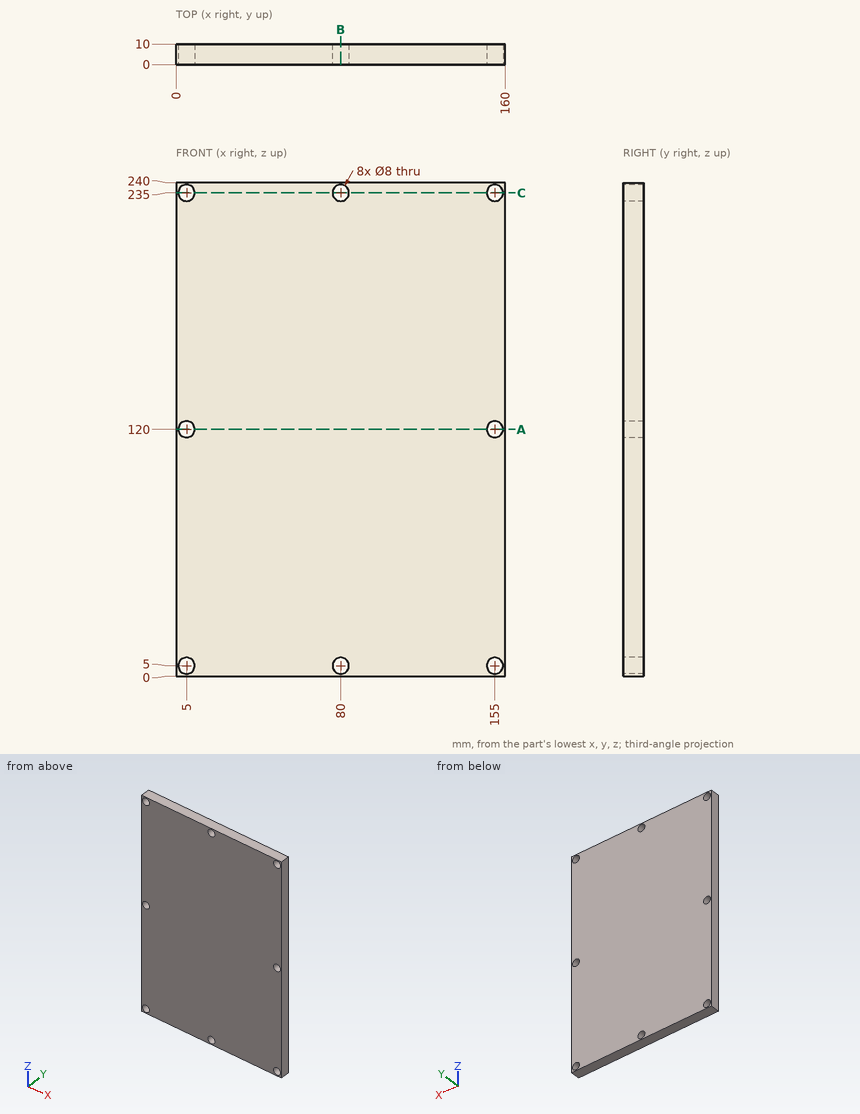
Print and shaded views of the part. All mm, measured from the part's lowest x, y and z. Coordinates: 2 decimals unless noted, no trailing zeros. Write each loop counter-clockwise with the first axis right and the second up, starting at its lowest first coordinate (ties: lowest second). Pieces come first, ordered by that corner, then holes. Notation, with made-up numbers: M -12,-11 L 4,-11 A37 ccw 4,26 Z; hole C 34,9 d11. An arc over 180 degrees is marked long. Return JSON: item names as keys, results as strings.
1. Saw through at A-A, the plane z = 120. Write the cut outline in (x, y), then the cut area to 3 significant figures.
Determined:
{"outline": "M 0,0 L 1,0 L 1,10 L 0,10 Z; M 9,0 L 151,0 L 151,10 L 9,10 Z; M 159,0 L 160,0 L 160,10 L 159,10 Z", "area": "1,440 mm²"}
2. Probe L1, parallel to Z at x = 155, y = 4.5; L2, parallel to X at y = 4.25, z = 120; L3, parallel to Z at x = 80, y = 4.5. List the from-to ranges inside material, lowest first.
Determined:
{"L1": "0 to 1, 9 to 116, 124 to 231, 239 to 240", "L2": "0 to 1, 9 to 151, 159 to 160", "L3": "0 to 1, 9 to 231, 239 to 240"}
3. Saw through at B-B, the plane x = 80. Write the cut outline in (y, z).
Determined:
{"outline": "M 0,0 L 10,0 L 10,1 L 0,1 Z; M 0,9 L 10,9 L 10,231 L 0,231 Z; M 0,239 L 10,239 L 10,240 L 0,240 Z"}
4. Saw through at C-C, the plane z = 235. Write the cut outline in (x, y).
Determined:
{"outline": "M 0,0 L 1,0 L 1,10 L 0,10 Z; M 9,0 L 76,0 L 76,10 L 9,10 Z; M 84,0 L 151,0 L 151,10 L 84,10 Z; M 159,0 L 160,0 L 160,10 L 159,10 Z"}
